```python
from build123d import *

# Parameters (mm, degrees)
SKETCH1_R             = 3.9624
SKETCH1_R_2           = 2.2352
BOSS_EXTRUDE1_DEPTH   = 5.5626
BOSS_EXTRUDE1_2_DEPTH = 5.5626
SKETCH2_R             = 3.9624
BOSS_EXTRUDE2_DEPTH   = 1.6002


with BuildPart() as part:
    # Sketch1 → Boss-Extrude1 (new body, symmetric)
    with BuildSketch(Plane.XY):
        with Locations((-5.9944, 0)):
            Circle(SKETCH1_R)
        with Locations((-5.9944, 0)):
            Circle(SKETCH1_R_2, mode=Mode.SUBTRACT)
    extrude(amount=BOSS_EXTRUDE1_DEPTH, both=True)



with BuildPart() as body_2:
    # Sketch1 → Boss-Extrude1 2 (new body, symmetric)
    with BuildSketch(Plane.XY):
        with Locations((5.9944, 0)):
            Circle(SKETCH1_R)
        with Locations((5.9944, 0)):
            Circle(SKETCH1_R_2, mode=Mode.SUBTRACT)
    extrude(amount=BOSS_EXTRUDE1_2_DEPTH, both=True)


with BuildPart() as part_1:
    add(part.part)

    add(body_2.part)  # Boss-Extrude2 merges body 2
    # Sketch2 → Boss-Extrude2 (add)
    with BuildSketch(Plane.XY.offset(5.5626)):
        with BuildLine():
            ThreePointArc((-2.074984615, 4.6024587), (-12.0396, 0), (-2.074984615, -4.6024587))
            ThreePointArc((-2.074984615, -4.6024587), (0, -3.838654482), (2.074984615, -4.6024587))
            ThreePointArc((2.074984615, -4.6024587), (12.0396, 0), (2.074984615, 4.6024587))
            ThreePointArc((2.074984615, 4.6024587), (0, 3.838654482), (-2.074984615, 4.6024587))
        make_face()
        with Locations((5.9944, 0)):
            Circle(SKETCH2_R, mode=Mode.SUBTRACT)
        with Locations((-5.9944, 0)):
            Circle(SKETCH2_R, mode=Mode.SUBTRACT)
    boss_extrude2 = extrude(amount=-BOSS_EXTRUDE2_DEPTH)

    # Mirror1: Boss-Extrude2 across plane
    add(boss_extrude2.mirror(Plane.XY))


solid = part_1.part
```
Geometry check sheet. Reference: the model listing, model coordinates, mm. A direction names the side the tool comes from. Give positions to 0.01 mm unless a question says otherwise; leave off trailing zeros. Order: outer loops, then holes, each group sorted by start corner. A loop starts at its lowest first (then second) coordinate and runs counter-clockwise, first axis right, second up. Notation, with made-up numbers: (88.5, -18) -> (96.5, -18) arc R11 ccw to (96.5, -2) -> close; hole circle Ø10 at (-23.5, 42). An arc over 180 degrees is marked (long way). Write each question's results on one line, items separated by ' | '. Start each with the question number.
(1) Sectioned sample at B-B (z = 1.75). Enter the section's corners in (x, y).
(2) Sectioned sample at C-C (x = 6). Enter the section's corners in (y, z).
(3) Gauge pin test, flat ends, axial feed: P1, Ø1, axis at y = -0.5, z = 1, coming from the -X side; P2, Ø1.5, axis at x = 4, z = -1, coming from the -Y side; P3, Ø3.5, axis at x = 5.99, y = 0, coming from the +Z side; P4, Ø4, axis at y = 3.5, z = 2.5, coming from the +X side. Record the tip position at first contact, or that the pin passes through.
(4) Sectioned sample at A-A (y = 0). Enter the section's corners in (x, z), plus the area to 3 significant figures.
(5) Mould release check, pull along X, two halves, no side actions. Record for faces 3 (the face through (12.037, -0.193, -4.774)), 4 (the face through (0, 0, -5.563)): pulls with the +X half, pulls with the -X half, needs draft (parallel to the pull), parting line crosses it, or undercut.
(6) Access from +Z, -Z, +X, -X, +Y, -Y to the whole of each face (thin tool, end or side, straight path). Record for faces 1 (the face through (0, 0, -3.962)), 2 (the face through (0.03, 3.84, -4.77)).
(7) Sectioned sample at D-D (y = -5). Enter the section's corners in (x, z), plus the area to 3 significant figures.
(8) Scan lines: line 1 (Z direction, x = 5.5, y = 5); line 2 (X direction, y = -1, z = -4.5); line 3 (X direction, y = 0.5, z = -3.75). Record each from-to range of solid material in increasing order.
Answer below:
1) outline: circle Ø7.92 at (-5.99, 0); circle Ø7.92 at (5.99, 0); hole circle Ø4.47 at (-5.99, 0); hole circle Ø4.47 at (5.99, 0)
2) outline: (-6.05, -5.56) -> (-2.24, -5.56) -> (-2.24, 5.56) -> (-6.05, 5.56) -> (-6.05, 3.96) -> (-3.96, 3.96) -> (-3.96, -3.96) -> (-6.05, -3.96) -> close; (2.24, -5.56) -> (6.05, -5.56) -> (6.05, -3.96) -> (3.96, -3.96) -> (3.96, 3.96) -> (6.05, 3.96) -> (6.05, 5.56) -> (2.24, 5.56) -> close
3) P1: x = -9.96 | P2: y = -3.76 | P3: through | P4: x = 11.65
4) outline: (-12.04, -5.56) -> (-8.23, -5.56) -> (-8.23, 5.56) -> (-12.04, 5.56) -> (-12.04, 3.96) -> (-9.96, 3.96) -> (-9.96, -3.96) -> (-12.04, -3.96) -> close; (-3.76, -5.56) -> (3.76, -5.56) -> (3.76, 5.56) -> (-3.76, 5.56) -> close; (8.23, -5.56) -> (12.04, -5.56) -> (12.04, -3.96) -> (9.96, -3.96) -> (9.96, 3.96) -> (12.04, 3.96) -> (12.04, 5.56) -> (8.23, 5.56) -> close; hole (-2.03, -3.96) -> (2.03, -3.96) -> (2.03, 3.96) -> (-2.03, 3.96) -> close | area: 103 mm2
5) face 3: undercut | face 4: needs draft
6) face 1: none | face 2: +Z, -Z, +Y
7) outline: (-9.39, -5.56) -> (-2.6, -5.56) -> (-2.6, -3.96) -> (-9.39, -3.96) -> close; (-9.39, 3.96) -> (-2.6, 3.96) -> (-2.6, 5.56) -> (-9.39, 5.56) -> close; (2.6, -5.56) -> (9.39, -5.56) -> (9.39, -3.96) -> (2.6, -3.96) -> close; (2.6, 3.96) -> (9.39, 3.96) -> (9.39, 5.56) -> (2.6, 5.56) -> close | area: 43.5 mm2
8) line 1: -5.56 to -3.96, 3.96 to 5.56 | line 2: -11.96 to -7.99, -4 to 4, 7.99 to 11.96 | line 3: -9.93 to -8.17, -3.82 to -2.06, 2.06 to 3.82, 8.17 to 9.93
